from build123d import *

# Parameters (mm, degrees)
F0_W     = 130.9254616499
F0_H     = 78.3314704895
F1_DEPTH = 25.4
F2_R     = 22.4537347063
F3_DEPTH = 45.466
F5_DEPTH = 38.1


with BuildPart() as f1:
    # F0 (on Top) → F1 (new body)
    with BuildSketch(Plane.XY):
        Rectangle(F0_W, F0_H)
    extrude(amount=F1_DEPTH)

    # F2 (on face) → F3 (join)
    with BuildSketch(Plane.XY.offset(25.4)):
        Circle(F2_R)
    extrude(amount=F3_DEPTH)

    # F4 (on Right) → F5 (cut, symmetric)
    with BuildSketch(Plane.YZ):
        Polygon((39.7252477705, 72.1768513322), (-29.9338120967, 71.8970969319), (39.7252477705, 40.2847565711), align=None)
    extrude(amount=F5_DEPTH, both=True, mode=Mode.SUBTRACT)


solid = f1.part
Read the model definition and answer for the solid it produces. Units are mm, in the model's axes. A direction names the side the tool comes from. Coordinates: 2 decimals unless noted, no trailing zeros. Loops run counter-clockwise (first coordinate to the right, second up) from the corner with the lowest first, then second, coordinate; pieces in that order, holes last. Notation, with made-up numbers: (55, 72.5) -> (87, 72.5) arc R25 cw to (87, 89.5) -> close; hole circle Ø3 at (-14, -25.75). An arc over 180 degrees is marked (long way). Answer in a Markdown table with one row per item.
Item 1: A cutting plane is placed at D-D on y = -31.5. Determine the outline of the cut face in (x, z), plus the area to 3 significant figures.
Returned:
| item | result |
|---|---|
| outline | (-65.46, 0) -> (65.46, 0) -> (65.46, 25.4) -> (-65.46, 25.4) -> close |
| area | 3,330 mm^2 |
Item 2: Each of these flat-tipped pins is pushed along its axis until it touches: P1, Ø10, axis at x = 49.5, y = -8, coming from the +Z side; P2, Ø6, axis at y = -11.5, z = 59.5, coming from the -X side; P3, Ø8, axis at x = -4, y = 24.5, coming from the -Z side; P4, Ø1.5, axis at y = 7, z = 49, coming from the -X side. Where does it stop, or does it pass through?
Returned:
| item | result |
|---|---|
| P1 | stops at z = 25.4 |
| P2 | stops at x = -20.78 |
| P3 | stops at z = 0 |
| P4 | stops at x = -21.57 |
Item 3: For faces 1 (the flat face through (-1, -39.166, 13)), 2 (the cylindrical face through (-4.87, -21.92, 41.86)), determine the directions among +Z, -Z, +X, -X, +Y, -Y from which every point of the face is accessible in a straight line to the end or side of a thin tool.
Returned:
| item | result |
|---|---|
| face 1 | +Z, -Z, +X, -X, -Y |
| face 2 | +Z |
Item 4: A cutting plane is placed at B-B on y = 2. Determine the outline of the cut face in (x, z), plus the area to 3 significant figures.
Returned:
| item | result |
|---|---|
| outline | (-65.46, 0) -> (65.46, 0) -> (65.46, 25.4) -> (22.36, 25.4) -> (22.36, 57.41) -> (-22.36, 57.41) -> (-22.36, 25.4) -> (-65.46, 25.4) -> close |
| area | 4,760 mm^2 |
Item 5: Straight lines are drawn through the part: line 1 along Z through (x, y) = (-39.5, -19); line 2 along X through (y, z) = (-19, 34); line 3 along X through (y, z) = (-12.5, 39). For each, find the intervals that lie inside material, in ascending order. Write a range as [from, to].
Returned:
| item | result |
|---|---|
| line 1 | z = [0, 25.4] |
| line 2 | x = [-11.97, 11.97] |
| line 3 | x = [-18.65, 18.65] |
Item 6: A cutting plane is placed at A-A on x = 0. Determine the outline of the cut face in (y, z), plus the area to 3 significant figures.
Returned:
| item | result |
|---|---|
| outline | (-39.17, 0) -> (39.17, 0) -> (39.17, 25.4) -> (22.45, 25.4) -> (22.45, 48.12) -> (-22.45, 68.5) -> (-22.45, 25.4) -> (-39.17, 25.4) -> close |
| area | 3,470 mm^2 |
Item 7: A cutting plane is placed at C-C on z = 39. Determine the outline of the cut face in (x, y).
Returned:
| item | result |
|---|---|
| outline | circle Ø44.91 at (0, 0) |
